from build123d import *

# Parameters (mm, degrees)
F0_W     = 101.6
F0_H     = 101.6
F1_DEPTH = 101.6
F2_R     = 25.4
F3_DEPTH = 101.6
F6_W     = 50.8
F6_H     = 50.8
F7_DEPTH = 101.6
F8_R     = 5.08


with BuildPart() as f1:
    # F0 (on Top) → F1 (new body)
    with BuildSketch(Plane.XY):
        Rectangle(F0_W, F0_H)
    extrude(amount=F1_DEPTH)

    # F2 (on face) → F3 (join)
    with BuildSketch(Plane.XY.offset(101.6)):
        Circle(F2_R)
    extrude(amount=F3_DEPTH)

    # F4 (on face) → F5 (revolve)
    with BuildSketch(Plane.XY.offset(203.2)):
        with BuildLine():
            Line((0, -25.4), (0, -38.1))
            ThreePointArc((0, -38.1), (38.1, 0), (0, 38.1))
            Line((0, 38.1), (0, 25.4))
            ThreePointArc((0, 25.4), (17.9605122421, 17.9605122421), (25.4, 0))
            ThreePointArc((25.4, 0), (17.9605122421, -17.9605122421), (0, -25.4))
        make_face()
        with BuildLine():
            Line((0, 25.4), (0, -25.4))
            ThreePointArc((0, -25.4), (17.9605122421, -17.9605122421), (25.4, 0))
            ThreePointArc((25.4, 0), (17.9605122421, 17.9605122421), (0, 25.4))
        make_face()
    revolve(axis=Axis((0, 0, 203.2), (0, -1, 0)))

    # F6 (on face) → F7 (cut)
    with BuildSketch(Plane.XZ.offset(50.8)):
        with Locations((0, 50.8)):
            Rectangle(F6_W, F6_H)
    extrude(amount=-F7_DEPTH, mode=Mode.SUBTRACT)

    # F8
    f8_edges = [f1.edges().sort_by_distance(p)[0] for p in [
        (50.8, 0, 101.6),
        (0, 50.8, 101.6),
        (0, -50.8, 101.6),
        (-50.8, 0, 101.6),
        (50.8, -50.8, 50.8),
        (50.8, 50.8, 50.8),
        (0, -50.8, 0),
        (-50.8, -50.8, 50.8),
        (-50.8, 0, 0),
        (0, 50.8, 0),
        (-50.8, 50.8, 50.8),
        (-25.4, 0, 101.6),
        (-25.4, 0, 174.801937),
    ]]
    fillet(f8_edges, radius=F8_R)


solid = f1.part
Input: part model. Units: mm. Frame: model coordinates. A direction names the side the tool comes from. Round coordinates to 2 decimals unless told otherwise and drop trailing zeros. Order: outer loops, then holes, each group sorted by start corner. A loop starts at its lowest first (then second) coordinate and runs counter-clockwise, first axis right, second up. Notation, with made-up numbers: (75, 50) - (97, 50) arc R17 ccw to (97, 65) - close; hole circle Ø10 at (81, -38.5). An arc over 180 degrees is marked (long way). Use a Markdown table: item, result.
1. Mould query, pull axis X, two halves, no side actions, for faces 1 (the face through (-1, 50.8, 81)), 2 (the face through (0, -1, 25.4)), 3 (the face through (50.8, -1, 48)). Classes: +X half, -X half, draft (parallel to the pull), parting line (faces both ways), or undercut.
Evaluation:
| item | result |
|---|---|
| face 1 | draft |
| face 2 | undercut |
| face 3 | +X half |
2. Section B-B on z = 119. Return the cut outline in (x, y).
Evaluation:
| item | result |
|---|---|
| outline | circle Ø50.8 at (0, 0) |
3. Material intervals for probe 1 along X at (y, z) = (33, 62); probe 2 along Z at (x, y) = (-20, 29.5); probe 3 along Z at (x, y) = (-41.5, 36), sorted ascending.
Evaluation:
| item | result |
|---|---|
| probe 1 | -50.8 to -25.4, 25.4 to 50.8 |
| probe 2 | 0 to 25.4, 76.2 to 101.6, 189.73 to 216.67 |
| probe 3 | 0 to 101.6 |
4. Access query for faces 4 (the face through (-1, 31, 101.6)), 5 (the face through (25.4, -1, 50)), 6 (the face through (2, 1, 0)). Directions: +Z, -Z, +X, -X, +Y, -Y. A direction counts if a zero-diameter tool reaches every point of the face in a straight line with its end or side. Return the directions, or none.
Evaluation:
| item | result |
|---|---|
| face 4 | none |
| face 5 | +Y, -Y |
| face 6 | -Z, +X, -X, +Y, -Y |
5. Section A-A on y = 43. Return the cut outline in (x, z).
Evaluation:
| item | result |
|---|---|
| outline | (-50.8, 5.08) arc R5.08 ccw to (-45.72, 0) - (50.8, 0) - (50.8, 96.52) arc R5.08 ccw to (45.72, 101.6) - (-45.72, 101.6) arc R5.08 ccw to (-50.8, 96.52) - close; hole (-25.4, 25.4) - (25.4, 25.4) - (25.4, 76.2) - (-25.4, 76.2) - close |
6. First-contact query: pin 1 (8 mm diameter, centred on x = 37, y = -24, fed in from +Z); pin 2 (6 mm diameter, centred on y = -4, z = 117.5, fed in from -X); pin 3 (10 mm diameter, centred on x = -24, z = 173, fed in from -Y). Flat tips, straight axial feed; report the tip coordinate or a pass-through.
Evaluation:
| item | result |
|---|---|
| pin 1 | z = 101.6 |
| pin 2 | x = -25.38 |
| pin 3 | y = -18.01 |
